Work out the finished part from the listing and answer in its coordinate system (mm). A direction names the side the tool comes from. Give positions to 0.01 mm unless a question says otherwise; leave off trailing zeros. Loops run counter-clockwise (first coordinate to the right, second up) from the corner with the lowest first, then second, coordinate; pieces in that order, holes last. Notation, with made-up numbers: M -34.75,82 L 21.25,82 A26 cw 21.25,118 Z; hole C 39.25,33.5 d10. An arc over 180 degrees is marked long. Use a Markdown table: item, result.
```python
from build123d import *

# Parameters (mm, degrees)
F1_DEPTH = 36
F2_R     = 2.2
F3_DEPTH = 12.0112263536
F2_R_2   = 3
F4_DEPTH = 1
F5_R     = 2.2
F6_DEPTH = 12.0112263536
F5_R_2   = 3
F7_DEPTH = 1


with BuildPart() as f1:
    # F0 (on Front) → F1 (new body)
    with BuildSketch(Plane.XZ):
        Polygon((-12, -21.1726237282), (-38.344139459, -30.7611063387), (-37.3180790291, -33.580184201), (-12, -24.3651570457), (13.3180790291, -33.580184201), (14.344139459, -30.7611063387), align=None)
    extrude(amount=F1_DEPTH)

    # F2 (on face) → F3 (cut, through all)
    with BuildSketch(Plane(origin=(6.4270771872, 0, -17.658249445), x_dir=(0.9396926208, 0, 0.3420201433), z_dir=(0.3420201433, 0, -0.9396926208))):
        with Locations((-40.5526228989, 27)):
            Circle(F2_R)
        with Locations((-28.5526228989, 27)):
            Circle(F2_R)
        with Locations((-28.5526228989, 9)):
            Circle(F2_R)
        with Locations((-40.5526228989, 9)):
            Circle(F2_R)
    extrude(amount=-F3_DEPTH, mode=Mode.SUBTRACT)

    # F2 (on face) → F4 (cut)
    with BuildSketch(Plane(origin=(6.4270771872, 0, -17.658249445), x_dir=(0.9396926208, 0, 0.3420201433), z_dir=(0.3420201433, 0, -0.9396926208))):
        with Locations((-40.5526228989, 27)):
            Circle(F2_R_2)
        with Locations((-40.5526228989, 27)):
            Circle(F2_R, mode=Mode.SUBTRACT)
        with Locations((-40.5526228989, 9)):
            Circle(F2_R_2)
        with Locations((-40.5526228989, 9)):
            Circle(F2_R, mode=Mode.SUBTRACT)
        with Locations((-28.5526228989, 9)):
            Circle(F2_R_2)
        with Locations((-28.5526228989, 9)):
            Circle(F2_R, mode=Mode.SUBTRACT)
        with Locations((-28.5526228989, 27)):
            Circle(F2_R_2)
        with Locations((-28.5526228989, 27)):
            Circle(F2_R, mode=Mode.SUBTRACT)
    extrude(amount=-F4_DEPTH, mode=Mode.SUBTRACT)

    # F5 (on face) → F6 (cut, through all)
    with BuildSketch(Plane(origin=(-9.2345438698, 0, -25.3717007612), x_dir=(0.9396926208, 0, -0.3420201433), z_dir=(-0.3420201433, 0, -0.9396926208))):
        with Locations((6, 27)):
            Circle(F5_R)
        with Locations((18, 27)):
            Circle(F5_R)
        with Locations((6, 9)):
            Circle(F5_R)
        with Locations((18, 9)):
            Circle(F5_R)
    extrude(amount=-F6_DEPTH, mode=Mode.SUBTRACT)

    # F5 (on face) → F7 (cut)
    with BuildSketch(Plane(origin=(-9.2345438698, 0, -25.3717007612), x_dir=(0.9396926208, 0, -0.3420201433), z_dir=(-0.3420201433, 0, -0.9396926208))):
        with Locations((6, 27)):
            Circle(F5_R_2)
        with Locations((6, 27)):
            Circle(F5_R, mode=Mode.SUBTRACT)
        with Locations((18, 27)):
            Circle(F5_R_2)
        with Locations((18, 27)):
            Circle(F5_R, mode=Mode.SUBTRACT)
        with Locations((18, 9)):
            Circle(F5_R_2)
        with Locations((18, 9)):
            Circle(F5_R, mode=Mode.SUBTRACT)
        with Locations((6, 9)):
            Circle(F5_R_2)
        with Locations((6, 9)):
            Circle(F5_R, mode=Mode.SUBTRACT)
    extrude(amount=-F7_DEPTH, mode=Mode.SUBTRACT)


solid = f1.part
```
(1) The mould has two halves that part along Z. Classify faces 3 (the cylindrical face through (-34.665, -9.132, -32.09)), 4 (the flat face through (-12, 0, -24)), 5 (the flat face through (0.482, -17.748, -28.908)): released by +Z, released by -Z, zero draft, split by the parting line, or undercut.
Entries:
| item | result |
|---|---|
| face 3 | undercut |
| face 4 | zero draft |
| face 5 | released by -Z |
(2) A cutting plane is placed at C-C (z = -22.25). Write down the section's boundary in (x, y).
Entries:
| item | result |
|---|---|
| outline | M -14.96,-36 L -9.04,-36 L -9.04,0 L -14.96,0 Z |
(3) Given P1, Ø5, axis at y = -21.5, z = -32, coming from the -X side; P2, Ø1.5, axis at x = -8, y = -19, coming from the +Z side; P3, Ø12, axis at x = -7.5, y = -4, coming from the -Z side, each flat-ended and moving along its own axis, determine where each tip first touches the part or whether it passes through.
Entries:
| item | result |
|---|---|
| P1 | stops at x = -38.34 |
| P2 | stops at z = -22.36 |
| P3 | stops at z = -28.19 |
(4) Which of the six approach directions +Z, -Z, +X, -X, +Y, -Y give full straight-line access (tool end or side, diameter ignored) to faces 1 (the flat face through (-24.84, -17.75, -29.04)), 2 (the cylindrical face through (-1.81, -10.86, -25.96))?
Entries:
| item | result |
|---|---|
| face 1 | -Z, +Y, -Y |
| face 2 | none |
(5) A cutting plane is placed at B-B (x = -22). Count the separate pieces of the cut face and the enclosed holes in it, and give its area (3 significant figures).
Entries:
| item | result |
|---|---|
| separate pieces | 3 |
| enclosed holes | 0 |
| area | 87.2 mm² |
(6) Consider probe 1 along Y at (x, z) = (6, -30.5); probe 2 along Y at (x, z) = (-5, -26.5); probe 3 along Z at (x, y) = (5, -15). Determine where each line is inside the solid, lowest interval first. Write a range as [from, to].
Entries:
| item | result |
|---|---|
| probe 1 | y = [-36, -29.3], [-24.7, -11.3], [-6.7, 0] |
| probe 2 | y = [-36, -29.52], [-24.48, -11.52], [-6.48, 0] |
| probe 3 | z = [-30.55, -27.36] |
(7) A cutting plane is placed at A-A (y = -4.5). Write down the section's boundary in (x, z).
Entries:
| item | result |
|---|---|
| outline | M -38.34,-30.76 L -37.32,-33.58 L -12,-24.37 L 13.32,-33.58 L 14.34,-30.76 L -12,-21.17 Z |
